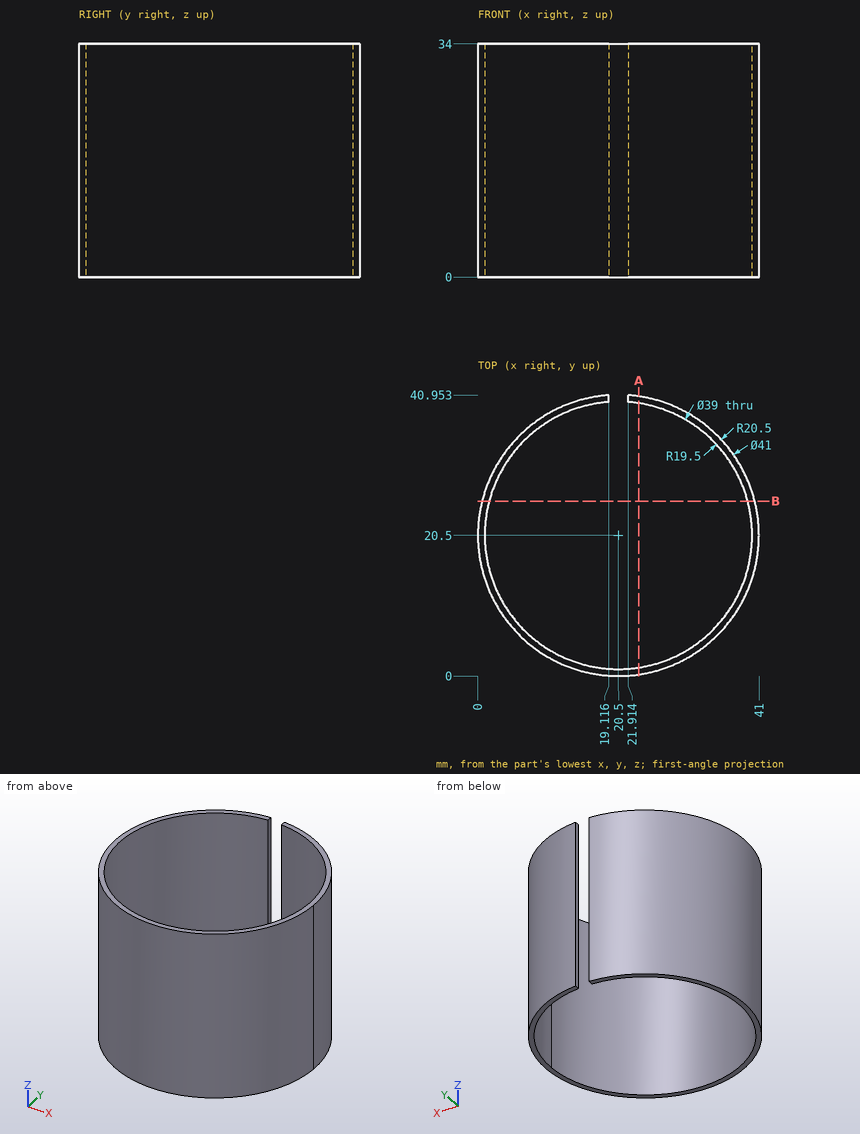
The figure shows three views and two pictorial views of one solid part (mm, origin at its lowest corner). Answer the questions. Round coordinates to 2 decimals unless told otherwise and drop trailing zeros. Write each loop counter-clockwise with the first axis right and the second up, starting at its lowest first coordinate (ties: lowest second). Pieces come first, ordered by that corner, then holes. Notation, with made-up numbers: (69, -27.75) - (122, -27.75) arc R13 ccw to (122, -15.75) - close; hole circle Ø2 at (-20.5, -33.5). An arc over 180 degrees is marked (long way). Use one line per item in the form item = value. Start each with the question number.
Item 1: Find the intervals of material crossed by line 1 (X direction, y = 20.5, z = 18); line 2 (Y direction, x = 20.5, z = 14.5); line 3 (Y direction, x = 28, z = 6), in increasing order. Write a range as [from, to].
Item 2: A cutting plane is placed at B-B (y = 25.5). Write down the section's boundary in (x, z).
Item 3: Flat-ended cylindrical pins translate along their axes: pin 1 Ø6 at (x, z) = (33, 10) entering from +Y (1 decimal); pin 2 Ø5 at (x, z) = (29.5, 12.5) entering from +Y; pin 3 Ø12 at (x, z) = (9.5, 22.5) entering from +Y. Find the tip coordinate at first contact, or state that the pin passes through.
Item 4: A cutting plane is placed at A-A (x = 23.5). Write down the section's boundary in (y, z).
The answers:
q1.line_1 = [0, 1], [40, 41]
q1.line_2 = [0, 1]
q1.line_3 = [1.42, 2.5], [38.5, 39.58]
q2.outline = (0.62, 0) - (1.65, 0) - (1.65, 34) - (0.62, 34) - close; (39.35, 0) - (40.38, 0) - (40.38, 34) - (39.35, 34) - close
q3.pin_1 = 38.7
q3.pin_2 = 39.94
q3.pin_3 = 40.38
q4.outline = (0.22, 0) - (1.23, 0) - (1.23, 34) - (0.22, 34) - close; (39.77, 0) - (40.78, 0) - (40.78, 34) - (39.77, 34) - close
